The model under review builds one solid part; all positions refer to its coordinate system, in mm. Face numbers are marked on the shaded views. A direction names the side the tool comes from. Round coordinates to 2 decimals unless told otherwise and drop trailing zeros. Write each loop counter-clockwise with the first axis right and the second up, starting at its lowest first coordinate (ties: lowest second). Pieces come first, ordered by that corner, then holes. Notation, with made-up numbers: (88, -23.75) -> (134, -23.75) arc R30 cw to (134, -1.75) -> close; hole circle Ø7 at (-4.75, 14.25). An arc over 180 degrees is marked (long way). Return JSON: item names as keys, results as strings. Group by question number.
1. Tool access review of the marked faces 1, 2, 3, 4 and 5: name each direction out of +Z, -Z, +X, -X, +Y, -Y from which nothing blocks a thin tool from reaching the whole face with its end or side.
2. Take a section at A-A, the plane z = 6. Write out the cut boundary in (x, y), then the cut area to 3 significant figures.
3. For line 1 along X through (y, z) = (-44.5, 10.5); line 2 along Y through (x, z) = (44.5, 12); line 3 along X through (y, z) = (-41, 24.5) (3 decimals), list the stretches that pass through material, from the lowest coordinate up. Write a range as from..to.
4. Take a section at B-B, the plane y = -20.5. Write out the cut boundary in (x, z).
5. Take a section at D-D, the plane y = -29. Write out the cut boundary in (x, z).
6. Take a section at C-C, the plane x = 27. Write out the cut boundary in (y, z), then the cut area to 3 significant figures.
7. Clearance check with flat-ended pins moving along their axes: P1, Ø10, axis at x = 9.5, z = 13.5, coming from the +Y side; P2, Ø6.5, axis at x = 43.5, z = 9, coming from the -Y side; P3, Ø6.5, axis at x = 44.5, z = 10, coming from the +Y side; P4, Ø5, axis at x = 14.5, y = -21.5, coming from the +Z side. State where each tip first meets the part, or that it passes through.
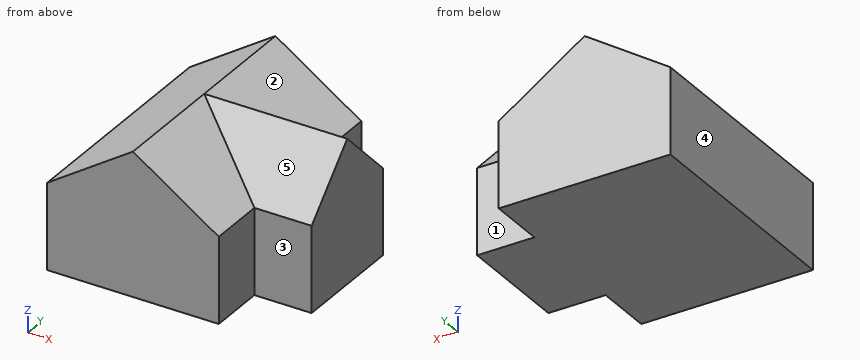
from build123d import *

# Parameters (mm, degrees)
F1_DEPTH = 50.8
F2_W     = 25.4
F2_H     = 31.75
F3_DEPTH = 12.7
F5_DEPTH = 50.8
F7_DEPTH = 12.7
F8_DEPTH = 31.75


with BuildPart() as f1:
    # F0 (on Front) → F1 (new body)
    with BuildSketch(Plane.XZ):
        Polygon((0, 19.05), (0, 0), (38.1, 0), (38.1, 19.05), (38.1, 31.75), (19.05, 31.75), align=None)
    extrude(amount=F1_DEPTH)

    # F2 (on face) → F3 (join)
    with BuildSketch(Plane.YZ.offset(38.1)):
        with Locations((-25.4, 15.875)):
            Rectangle(F2_W, F2_H)
    extrude(amount=F3_DEPTH)

    # F4 (on face) → F5 (cut)
    with BuildSketch(Plane.XZ.offset(50.8)):
        Polygon((38.1, 31.75), (19.05, 31.75), (38.1, 19.05), align=None)
    extrude(amount=-F5_DEPTH, mode=Mode.SUBTRACT)

    # F6 (on face) → F7 (cut)
    with BuildSketch(Plane.YZ.offset(50.8)):
        Polygon((-38.1, 31.75), (-38.1, 19.05), (-25.4, 31.75), align=None)
        Polygon((-12.7, 31.75), (-25.4, 31.75), (-12.7, 19.05), align=None)
    extrude(amount=-F7_DEPTH, mode=Mode.SUBTRACT)

    # F8 (add): a face of the model
    f8_faces = [f1.faces().sort_by_distance(p)[0] for p in [
        (50.8, -25.4, 12.9645833333),
    ]]
    extrude(f8_faces, amount=-F8_DEPTH)


solid = f1.part
Output:
{
 "1": {"face 1": "+Z, -Z, +X, +Y", "face 2": "+Z, +X, +Y", "face 3": "+Z, -Z, +X, -Y", "face 4": "+Z, -Z, -X, +Y, -Y", "face 5": "+Z, +X, -Y"},
 "2": {"outline": "(0, -50.8) -> (38.1, -50.8) -> (38.1, -38.1) -> (50.8, -38.1) -> (50.8, -12.7) -> (38.1, -12.7) -> (38.1, 0) -> (0, 0) -> close", "area": "2,260 mm^2"},
 "3": {"line 1": "x = 0..38.1", "line 2": "y = -38.1..-12.7", "line 3": "x = 8.175..29.925"},
 "4": {"outline": "(0, 0) -> (50.8, 0) -> (50.8, 26.85) -> (26.4, 26.85) -> (19.05, 31.75) -> (0, 19.05) -> close"},
 "5": {"outline": "(0, 0) -> (50.8, 0) -> (50.8, 28.15) -> (24.45, 28.15) -> (19.05, 31.75) -> (0, 19.05) -> close"},
 "6": {"outline": "(-50.8, 0) -> (0, 0) -> (0, 26.45) -> (-20.1, 26.45) -> (-25.4, 31.75) -> (-30.7, 26.45) -> (-50.8, 26.45) -> close", "area": "1,370 mm^2"},
 "7": {"P1": "stops at y = 0", "P2": "stops at y = -38.1", "P3": "stops at y = -12.7", "P4": "stops at z = 30.38"}
}
